```python
from build123d import *

# Parameters (mm, degrees)
EXTRUDE_1_DEPTH     = 3
SKETCH_2_R          = 1.55
SKETCH_2_R_2        = 11
SKETCH_2_R_3        = 1.25
SKETCH_2_R_4        = 5
SKETCH_2_R_5        = 1.6
CUT_EXTRUDE_1_DEPTH = 130.55693729
EXTRUDE_START       = -3
EXTRUDE_2_DEPTH     = 3
SKETCH_3_R          = 1.5
SKETCH_3_R_2        = 1.6
SKETCH_3_W          = 46
SKETCH_3_H          = 5
CUT_EXTRUDE_2_DEPTH = 135.433749111
SKETCH_5_R          = 1
CUT_EXTRUDE_3_DEPTH = 135.433749111
SKETCH_6_R          = 3
SKETCH_6_R_2        = 1.025
CUT_EXTRUDE_4_DEPTH = 135.433749111
SKETCH_7_W          = 14
SKETCH_7_H          = 9
CUT_EXTRUDE_5_DEPTH = 135.433749111
FILLET_1_R          = 2


with BuildPart() as part:
    # ｽｹｯﾁ1 → ﾎﾞｽ - 押し出し1 (new body)
    with BuildSketch(Plane.XY):
        with BuildLine():
            Line((-96, 30), (96, 30))
            ThreePointArc((96, 30), (126, 0), (96, -30))
            Line((96, -30), (-96, -30))
            ThreePointArc((-96, -30), (-126, 0), (-96, 30))
        make_face()
    extrude(amount=EXTRUDE_1_DEPTH)

    # ｽｹｯﾁ2 → ｶｯﾄ - 押し出し1 (cut, through all)
    with BuildSketch(Plane.XY.offset(3)):
        with Locations((-24.362267564, 4.80144627)):
            Circle(SKETCH_2_R)
        with Locations((-56, 0)):
            Circle(SKETCH_2_R)
        with Locations((-96, 0)):
            Circle(SKETCH_2_R_2)
        with Locations(Location((24.362267564, 4.80144627, 0), (0, 0, 180))):
            Circle(SKETCH_2_R)
        with Locations(Location((56, 0, 0), (0, 0, 180))):
            Circle(SKETCH_2_R)
        with Locations(Location((96, 0, 0), (0, 0, 180))):
            Circle(SKETCH_2_R_2)
        with Locations((-76, 27)):
            Circle(SKETCH_2_R_3)
        with Locations((-76, -27)):
            Circle(SKETCH_2_R_3)
        with Locations(Location((76, 27, 0), (0, 0, 180))):
            Circle(SKETCH_2_R_3)
        with Locations(Location((76, -27, 0), (0, 0, 180))):
            Circle(SKETCH_2_R_3)
        with Locations((0, -9)):
            Circle(SKETCH_2_R_4)
        with Locations((-69, 25)):
            Circle(SKETCH_2_R_5)
        with Locations(Location((-69, -25, 0), (0, 0, 180))):
            Circle(SKETCH_2_R_5)
        with Locations((69, -25)):
            Circle(SKETCH_2_R_5)
        with Locations(Location((69, 25, 0), (0, 0, 180))):
            Circle(SKETCH_2_R_5)
    extrude(amount=-CUT_EXTRUDE_1_DEPTH, mode=Mode.SUBTRACT)

    # ｽｹｯﾁ4 → ﾎﾞｽ - 押し出し2 (add)
    with BuildSketch(Plane.XY.offset(3).offset(EXTRUDE_START)):
        with BuildLine():
            Line((-124.26065672, 10.06654269), (-120.611311687, 20.311657664))
            ThreePointArc((-120.611311687, 20.311657664), (-106.051810297, 39.489926307), (-83.1, 46.77))
            Line((-83.1, 46.77), (83.1, 46.77))
            ThreePointArc((83.1, 46.77), (106.051810297, 39.489926307), (120.611311687, 20.311657664))
            Line((120.611311687, 20.311657664), (124.26065672, 10.06654269))
            ThreePointArc((124.26065672, 10.06654269), (113.291670239, 24.515263416), (96, 30))
            Line((96, 30), (-96, 30))
            ThreePointArc((-96, 30), (-113.291670239, 24.515263416), (-124.26065672, 10.06654269))
        make_face()
        with BuildLine():
            Line((-84.297970262, -31.75), (84.297970262, -31.75))
            ThreePointArc((84.297970262, -31.75), (94.651109882, -30.980141557), (104.776522304, -28.6875))
            ThreePointArc((104.776522304, -28.6875), (100.437059837, -29.670060667), (96, -30))
            Line((96, -30), (-96, -30))
            ThreePointArc((-96, -30), (-100.437059837, -29.670060667), (-104.776522304, -28.6875))
            ThreePointArc((-104.776522304, -28.6875), (-94.651109882, -30.980141557), (-84.297970262, -31.75))
        make_face()
    extrude(amount=EXTRUDE_2_DEPTH)

    # ｽｹｯﾁ3 → ｶｯﾄ - 押し出し2 (cut, through all)
    with BuildSketch(Plane.XY.offset(3)):
        with Locations((-61.057299255, 37.02)):
            Circle(SKETCH_3_R)
        with Locations(Location((-9.057299255, 37.02, 0), (0, 0, 180))):
            Circle(SKETCH_3_R)
        with Locations((9.057299255, 37.02)):
            Circle(SKETCH_3_R)
        with Locations(Location((61.057299255, 37.02, 0), (0, 0, 180))):
            Circle(SKETCH_3_R)
        with Locations((-69, 35)):
            Circle(SKETCH_3_R_2)
        with Locations((61.057299255, -22)):
            Circle(SKETCH_3_R)
        with Locations(Location((9.057299255, -22, 0), (0, 0, 180))):
            Circle(SKETCH_3_R)
        with Locations((-9.057299255, -22)):
            Circle(SKETCH_3_R)
        with Locations(Location((-61.057299255, -22, 0), (0, 0, 180))):
            Circle(SKETCH_3_R)
        with Locations(Location((69, 35, 0), (0, 0, 180))):
            Circle(SKETCH_3_R_2)
        with Locations((-35.057299255, 37.02)):
            Rectangle(SKETCH_3_W, SKETCH_3_H)
        with Locations((35.057299255, 37.02)):
            Rectangle(SKETCH_3_W, SKETCH_3_H)
        with Locations((35.057299255, -22)):
            Rectangle(SKETCH_3_W, SKETCH_3_H)
        with Locations((-35.057299255, -22)):
            Rectangle(SKETCH_3_W, SKETCH_3_H)
    extrude(amount=-CUT_EXTRUDE_2_DEPTH, mode=Mode.SUBTRACT)

    # ｽｹｯﾁ5 → ｶｯﾄ - 押し出し3 (cut, through all)
    with BuildSketch(Plane.XY.offset(3)):
        with Locations((-58.057299255, 39.52)):
            Circle(SKETCH_5_R)
        with Locations((-58.057299255, 34.52)):
            Circle(SKETCH_5_R)
        with Locations((-12.057299255, 39.52)):
            Circle(SKETCH_5_R)
        with Locations((-12.057299255, 34.52)):
            Circle(SKETCH_5_R)
        with Locations((-12.057299255, -19.5)):
            Circle(SKETCH_5_R)
        with Locations((-12.057299255, -24.5)):
            Circle(SKETCH_5_R)
        with Locations((-58.057299255, -19.5)):
            Circle(SKETCH_5_R)
        with Locations((-58.057299255, -24.5)):
            Circle(SKETCH_5_R)
        with Locations((58.057299255, -24.5)):
            Circle(SKETCH_5_R)
        with Locations((58.057299255, -19.5)):
            Circle(SKETCH_5_R)
        with Locations((12.057299255, -24.5)):
            Circle(SKETCH_5_R)
        with Locations((12.057299255, -19.5)):
            Circle(SKETCH_5_R)
        with Locations((12.057299255, 34.52)):
            Circle(SKETCH_5_R)
        with Locations((12.057299255, 39.52)):
            Circle(SKETCH_5_R)
        with Locations((58.057299255, 34.52)):
            Circle(SKETCH_5_R)
        with Locations((58.057299255, 39.52)):
            Circle(SKETCH_5_R)
    extrude(amount=-CUT_EXTRUDE_3_DEPTH, mode=Mode.SUBTRACT)

    # ｽｹｯﾁ6 → ｶｯﾄ - 押し出し4 (cut, through all)
    with BuildSketch(Plane.XY.offset(3)):
        with Locations((-8.749968889, -0.143333333)):
            Circle(SKETCH_6_R)
        with Locations((0.587451619, 3.436132863)):
            Circle(SKETCH_6_R)
        with Locations((-12.990381057, -9.75)):
            Circle(SKETCH_6_R_2)
        with Locations((0, 12.75)):
            Circle(SKETCH_6_R_2)
        with Locations((12.990381057, -9.75)):
            Circle(SKETCH_6_R_2)
    extrude(amount=-CUT_EXTRUDE_4_DEPTH, mode=Mode.SUBTRACT)

    # ｽｹｯﾁ7 → ｶｯﾄ - 押し出し5 (cut, through all)
    with BuildSketch(Plane.XY.offset(3)):
        with Locations((-57.057299255, 27.02)):
            Rectangle(SKETCH_7_W, SKETCH_7_H)
        with Locations((57.057299255, 27.02)):
            Rectangle(SKETCH_7_W, SKETCH_7_H)
    extrude(amount=-CUT_EXTRUDE_5_DEPTH, mode=Mode.SUBTRACT)

    # ﾌｨﾚｯﾄ1
    fillet_1_edges = [part.edges().sort_by_distance(p)[0] for p in [
        (-64.057299255, 22.52, 1.5),
        (-64.057299255, 31.52, 1.5),
        (-50.057299255, 31.52, 1.5),
        (-50.057299255, 22.52, 1.5),
        (50.057299255, 22.52, 1.5),
        (50.057299255, 31.52, 1.5),
        (64.057299255, 31.52, 1.5),
        (64.057299255, 22.52, 1.5),
    ]]
    fillet(fillet_1_edges, radius=FILLET_1_R)


solid = part.part
```
The listing builds one solid part. Answer for the finished solid, in the listing's coordinates (mm). Coordinates: 2 decimals unless noted, no trailing zeros. Write each loop counter-clockwise with the first axis right and the second up, starting at its lowest first coordinate (ties: lowest second). Pieces come first, ordered by that corner, then holes.
Q1. Find the intervals of material crossed by line 1 along Y through (x, z) = (30.5, 0.4); line 2 along X through (y, z) = (7, 2.6); line 3 along Y through (x, z) = (25, 2.15), in increasing order.
Returned:
line 1: y = -31.75 to -24.5, -19.5 to 34.52, 39.52 to 46.77
line 2: x = -125.17 to -104.49, -87.51 to 87.51, 104.49 to 125.17
line 3: y = -31.75 to -24.5, -19.5 to 3.39, 6.21 to 34.52, 39.52 to 46.77
Q2. The mould has two halves that part along Y. Classify faces 1 (the flat face through (2, 8, 3)), 2 (the cylindrical face through (-0.651, -4.043, 1.521)), 3 (the cylindrical face through (-122.65, -13.78, 1.48)): released by +Y, released by -Y, zero draft, split by the parting line, or undercut.
Returned:
face 1: zero draft
face 2: undercut
face 3: split by the parting line
Q3. Section A-A, the plane x = 39.5 is taken. Write down the section's boundary in (y, z), then the cut area to 3 significant figures.
Returned:
outline: (-31.75, 0) - (-24.5, 0) - (-24.5, 3) - (-31.75, 3) - close; (-19.5, 0) - (34.52, 0) - (34.52, 3) - (-19.5, 3) - close; (39.52, 0) - (46.77, 0) - (46.77, 3) - (39.52, 3) - close
area: 206 mm2
Q4. Given P1, Ø1.5, axis at x = -76, y = 27, coming from the +Z side; P2, Ø1.5, axis at y = -21.5, z = 1, coming from the +X side, each flat-ended and moving along its own axis, determine where each tip first touches the part or whether it passes through.
Returned:
P1: passes through
P2: stops at x = 117.67
Q5. Section B-B, the plane z = 1.9 is taken. Give the number of separate pieces and of enclosed holes in the cut face, then the cut area to 3 significant figures.
Returned:
separate pieces: 1
enclosed holes: 36
area: 16,100 mm2
